Build history of the part. All positions in model axes, mm. Face numbers are marked on the shaded views. Give positions to 0.01 mm unless a question says otherwise; leave off trailing zeros. Order: outer loops, then holes, each group sorted by start corner. A loop starts at its lowest first (then second) coordinate and runs counter-clockwise, first axis right, second up. Notation, with made-up numbers: (52, 18.25) - (80, 18.25) arc R26 ccw to (80, 36.25) - close; hole circle Ø1 at (85, -7). An arc over 180 degrees is marked (long way). Write each question's results on one line, items separated by ' | '. Start each with the question number.
1) Two-plate mould, pull along X, no slides. Class the marked faces 1, 2, 3 and 4: +X half, -X half, draft (parallel to the pull), parting line (faces both ways), or undercut.
2) Cut at B-B on z = 22.75. State how many separate pieces and enclosed holes the cut face has, plus the area to 3 significant figures.
3) Cut at D-D on x = 32.5. List the corners of the cut face in (y, z).
4) Cut at C-C on y = 16.5. List the corners of the cut face in (x, z), plus the area to 3 significant figures.
5) Cut at A-A on z = 6. List the corners of the cut face in (x, y).
6) Drill centre lines: line 1 along X through (y, z) = (10.5, 15); line 2 along Y through (x, z) = (49.5, 7); line 3 along X through (y, z) = (16.5, 24). Where is each one in solid material? Low to high. Write a range as from..to.
7) Drop flat-ended pins along their axis: pin 1 Ø1.5 at (x, y) = (58.5, 16.5) entering from +Z; pin 2 Ø2 at (x, z) = (53, 6.5) entering from -Y; pin 3 Ø2.5 at (x, y) = (11.5, 1.5) entering from +Z; pin 4 Ø1 at (x, y) = (105.5, 37) entering from +Z. Give the stop position or say it passes through.
from build123d import *

# Parameters (mm, degrees)
SKETCH1_W           = 106.9
SKETCH1_H           = 98.3
BOSS_EXTRUDE2_DEPTH = 3.2
SKETCH2_W           = 106.9
SKETCH2_H           = 98.3
SKETCH2_W_2         = 100.5
SKETCH2_H_2         = 91.9
BOSS_EXTRUDE3_DEPTH = 24
SKETCH3_W           = 3.2
SKETCH3_H           = 1
CUT_EXTRUDE1_DEPTH  = 24
SKETCH4_W           = 3.2
SKETCH4_H           = 31
CUT_EXTRUDE2_DEPTH  = 18
SKETCH5_W           = 91.9
SKETCH5_H           = 3.2
CUT_EXTRUDE3_DEPTH  = 18
SKETCH6_W           = 3.2
SKETCH6_H           = 34.9
CUT_EXTRUDE4_DEPTH  = 19
SKETCH7_W           = 9
SKETCH7_H           = 3.2
CUT_EXTRUDE5_DEPTH  = 18


with BuildPart() as part:
    # Sketch1 → Boss-Extrude2 (new body)
    with BuildSketch(Plane.XY):
        with Locations((53.45, 49.15)):
            Rectangle(SKETCH1_W, SKETCH1_H)
    extrude(amount=BOSS_EXTRUDE2_DEPTH)

    # Sketch2 → Boss-Extrude3 (add)
    with BuildSketch(Plane.XY.offset(3.2)):
        with Locations((53.45, 49.15)):
            Rectangle(SKETCH2_W, SKETCH2_H)
        with Locations((53.45, 49.15)):
            Rectangle(SKETCH2_W_2, SKETCH2_H_2, mode=Mode.SUBTRACT)
    extrude(amount=BOSS_EXTRUDE3_DEPTH)

    # Sketch3 → Cut-Extrude1 (cut)
    with BuildSketch(Plane.XY.offset(27.2)):
        with Locations((1.6, 94.6)):
            Rectangle(SKETCH3_W, SKETCH3_H)
        with Locations((105.3, 94.6)):
            Rectangle(SKETCH3_W, SKETCH3_H)
        with Locations((105.3, 3.7)):
            Rectangle(SKETCH3_W, SKETCH3_H)
        with Locations((1.6, 3.7)):
            Rectangle(SKETCH3_W, SKETCH3_H)
    extrude(amount=-CUT_EXTRUDE1_DEPTH, mode=Mode.SUBTRACT)

    # Sketch4 → Cut-Extrude2 (cut)
    with BuildSketch(Plane.XY.offset(27.2)):
        with Locations((1.6, 35.6)):
            Rectangle(SKETCH4_W, SKETCH4_H)
    extrude(amount=-CUT_EXTRUDE2_DEPTH, mode=Mode.SUBTRACT)

    # Sketch5 → Cut-Extrude3 (cut)
    with BuildSketch(Plane.XY.offset(27.2)):
        with Locations((53.45, 96.7)):
            Rectangle(SKETCH5_W, SKETCH5_H)
    extrude(amount=-CUT_EXTRUDE3_DEPTH, mode=Mode.SUBTRACT)

    # Sketch6 → Cut-Extrude4 (cut)
    with BuildSketch(Plane.XY.offset(27.2)):
        with Locations((105.3, 31.65)):
            Rectangle(SKETCH6_W, SKETCH6_H)
    extrude(amount=-CUT_EXTRUDE4_DEPTH, mode=Mode.SUBTRACT)

    # Sketch7 → Cut-Extrude5 (cut)
    with BuildSketch(Plane.XY.offset(27.2)):
        with Locations((13.5, 1.6)):
            Rectangle(SKETCH7_W, SKETCH7_H)
    extrude(amount=-CUT_EXTRUDE5_DEPTH, mode=Mode.SUBTRACT)


solid = part.part
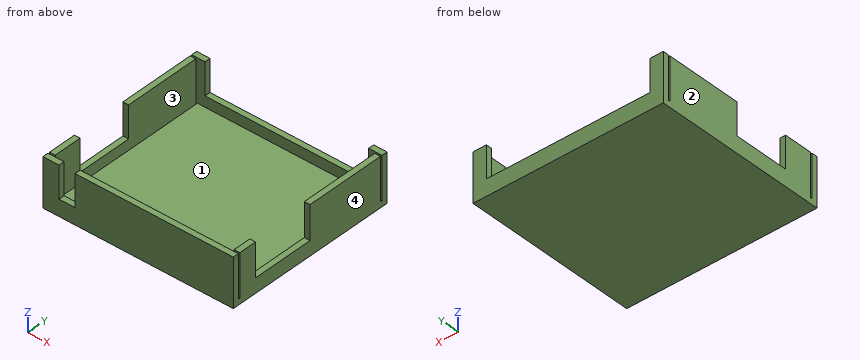
Results:
1) face 1: undercut | face 2: -X half | face 3: undercut | face 4: +X half
2) separate pieces: 8 | enclosed holes: 0 | area: 726 mm^2
3) outline: (0, 0) - (98.3, 0) - (98.3, 9.2) - (95.1, 9.2) - (95.1, 3.2) - (3.2, 3.2) - (3.2, 27.2) - (0, 27.2) - close
4) outline: (0, 0) - (106.9, 0) - (106.9, 8.2) - (103.7, 8.2) - (103.7, 3.2) - (3.2, 3.2) - (3.2, 27.2) - (0, 27.2) - close | area: 435 mm^2
5) outline: (0, 0) - (106.9, 0) - (106.9, 3.2) - (0, 3.2) - close; (0, 4.2) - (3.2, 4.2) - (3.2, 94.1) - (0, 94.1) - close; (0, 95.1) - (106.9, 95.1) - (106.9, 98.3) - (0, 98.3) - close; (103.7, 4.2) - (106.9, 4.2) - (106.9, 94.1) - (103.7, 94.1) - close
6) line 1: 0..3.2, 103.7..106.9 | line 2: 0..3.2, 95.1..98.3 | line 3: 0..3.2
7) pin 1: z = 3.2 | pin 2: y = 0 | pin 3: z = 9.2 | pin 4: z = 8.2
